from build123d import *

# Parameters (mm, degrees)
SKETCH1_W           = 406.4
SKETCH1_H           = 76.2
BOSS_EXTRUDE1_DEPTH = 25.4
SKETCH2_W           = 330.2
SKETCH2_H           = 50.8
CUT_EXTRUDE1_DEPTH  = 336.04901134
SKETCH3_W           = 330.2
SKETCH3_H           = 25.4
BOSS_EXTRUDE2_DEPTH = 88.9
SKETCH4_W           = 50.8
SKETCH4_H           = 25.4
CUT_EXTRUDE2_DEPTH  = 346.710702756
SKETCH5_W           = 304.8
SKETCH5_H           = 88.9
CUT_EXTRUDE3_DEPTH  = 358.635247144
HOLE1_D             = 12.7
HOLE1_DEPTH         = 3.302


with BuildPart() as part:
    # Sketch1 → Boss-Extrude1 (new body)
    with BuildSketch(Plane.XY.offset(25.4)):
        with Locations((127, -12.7)):
            Rectangle(SKETCH1_W, SKETCH1_H)
    extrude(amount=-BOSS_EXTRUDE1_DEPTH)

    # Sketch2 → Cut-Extrude1 (cut, through all)
    with BuildSketch(Plane(origin=(0, 0, 0), x_dir=(-1, 0, 0), z_dir=(0, 0, -1))):
        with Locations((-165.1, -25.4)):
            Rectangle(SKETCH2_W, SKETCH2_H)
    extrude(amount=-CUT_EXTRUDE1_DEPTH, mode=Mode.SUBTRACT)

    # Sketch3 → Boss-Extrude2 (add)
    with BuildSketch(Plane.XY.offset(25.4)):
        with Locations((165.1, 12.7)):
            Rectangle(SKETCH3_W, SKETCH3_H)
    extrude(amount=BOSS_EXTRUDE2_DEPTH)

    # Sketch4 → Cut-Extrude2 (cut, through all)
    with BuildSketch(Plane.XY.offset(25.4)):
        with Locations((-50.8, 12.7)):
            Rectangle(SKETCH4_W, SKETCH4_H)
    extrude(amount=-CUT_EXTRUDE2_DEPTH, mode=Mode.SUBTRACT)

    # Sketch5 → Cut-Extrude3 (cut, through all)
    with BuildSketch(Plane(origin=(0, 25.4, 0), x_dir=(-1, 0, 0), z_dir=(0, 1, 0))):
        with Locations((-177.8, 44.45)):
            Rectangle(SKETCH5_W, SKETCH5_H)
    extrude(amount=-CUT_EXTRUDE3_DEPTH, mode=Mode.SUBTRACT)

    # Hole1
    with Locations(Plane(origin=(0, 0, 0), x_dir=(-1, 0, 0), z_dir=(0, 0, -1))):
        with Locations((-12.7, 12.7)):
            Hole(HOLE1_D / 2, depth=HOLE1_DEPTH)


solid = part.part
Work out the finished part from the listing and answer in its coordinate system (mm). A direction names the side the tool comes from. Give positions to 0.01 mm unless a question says otherwise; leave off trailing zeros. Write each loop counter-clockwise with the first axis right and the second up, starting at its lowest first coordinate (ties: lowest second). Pieces come first, ordered by that corner, then holes. Notation, with made-up numbers: M -6.75,71 L 40.25,71 A21 cw 40.25,75 Z; hole C 72.5,-27.5 d7. An arc over 180 degrees is marked long. Answer as CSV lines item,"result".
Q1. A cutting plane is placed at A-A on y = 12.7. Write down the section's boundary in (x, z), plus the area to 3 significant figures.
A:
outline,"M -25.4,0 L 6.35,0 L 6.35,3.3 L 19.05,3.3 L 19.05,0 L 25.4,0 L 25.4,88.9 L 330.2,88.9 L 330.2,114.3 L 0,114.3 L 0,25.4 L -25.4,25.4 Z"
area,"11,200 mm²"
Q2. A cutting plane is placed at D-D on y = -18. Write down the section's boundary in (x, z), plus the area to 3 significant figures.
A:
outline,"M -76.2,0 L 0,0 L 0,25.4 L -76.2,25.4 Z"
area,"1,940 mm²"
Q3. A tool of negligible diameter and unlimited length cuts with its end or side. For faces 4 (the flat face through (-51, 0, 13)), 5 (the cylindrical face through (8.02, 16.99, 1.67)), 6 (the flat face through (180, 13, 88.9)), from which of +Z, -Z, +X, -X, +Y, -Y can it reach the whole face along a straight path? Write none if from no direction.
A:
face 4,"+Z, -Z, -X, +Y"
face 5,"-Z"
face 6,"-Z, +X, +Y, -Y"
Q4. The mould has two halves that part along Y. Classify faces 1 (the flat face through (-26, -21, 0)), 2 (the flat face through (13, 13, 3.302)), 3 (the flat face through (128, 0, 91)): +Y half, -Y half, draft (parallel to the pull), parting line (faces both ways), or undercut.
A:
face 1,"draft"
face 2,"undercut"
face 3,"-Y half"
Q5. A cutting plane is placed at B-B on x = 12.7. Write down the section's boundary in (y, z), plus the area to 3 significant figures.
A:
outline,"M 0,0 L 6.35,0 L 6.35,3.3 L 19.05,3.3 L 19.05,0 L 25.4,0 L 25.4,114.3 L 0,114.3 Z"
area,"2,860 mm²"
Q6. Given P1, Ø6.5, axis at x = 10.5, y = 11, coming from the -Z side; P2, Ø1.5, axis at x = 69.5, y = 9, coming from the -Z side; P3, Ø12, axis at y = -7.5, z = 51.5, coming from the -X side; P4, Ø12.5, axis at y = -14, z = 18.5, coming from the +X side, each flat-ended and moving along its own axis, determine where each tip first touches the part or whether it passes through.
A:
P1,"stops at z = 3.3"
P2,"stops at z = 88.9"
P3,"passes through"
P4,"stops at x = 0"
Q7. A cutting plane is placed at C-C on z = 56. Write down the section's boundary in (x, y).
A:
outline,"M 0,0 L 25.4,0 L 25.4,25.4 L 0,25.4 Z"
Q8. Find the intervals of material crossed by probe 1 along X at (y, z) = (12, 1); probe 2 along Y at (x, z) = (12.7, 1.2); probe 3 along Z at (x, y) = (285.5, 3.5), in increasing order. Write a range as [from, to].
A:
probe 1,"x = [-25.4, 6.39], [19.01, 25.4]"
probe 2,"y = [0, 6.35], [19.05, 25.4]"
probe 3,"z = [88.9, 114.3]"
